from build123d import *

# Parameters (mm, degrees)
F2_R = 5
F4_D = 11


with BuildPart() as f1:
    # F0 (on Front) → F1 (revolve)
    with BuildSketch(Plane.XZ):
        Polygon((0, 101), (0, 32), (10, 32), (10, 55), (32, 55), (32, 70), (20, 70), (20, 101), align=None)
    revolve(axis=Axis((86.927190423, 0, 0), (1, 0, 0)))

    # F2
    f2_edges = [f1.edges().sort_by_distance(p)[0] for p in [
        (20, 0, -70),
    ]]
    fillet(f2_edges, radius=F2_R)

    # F4 (through all)
    with Locations(Plane.YZ.offset(20)):
        with Locations((46.25, 80.1073498501), (-92.5, 0), (46.25, -80.1073498501)):
            Hole(F4_D / 2)


solid = f1.part
Source: CAD feature listing. Evaluate the final solid. Frame: model axes, mm. A direction names the side the tool comes from. Coordinates: 2 decimals unless noted, no trailing zeros. Loops run counter-clockwise (first coordinate to the right, second up) from the corner with the lowest first, then second, coordinate; pieces in that order, holes last. Notation, with made-up numbers: (-38.5, 52) - (-28.5, 52) arc R18 cw to (-28.5, 84) - close; hole circle Ø1 at (76, 35.25). An arc over 180 degrees is marked (long way). Return JSON: item names as keys, results as strings.
Q1. Section D-D, the plane x = 29.5. Return loops of the section in (y, z).
Results:
{"outline": "circle Ø140 at (0, 0); hole circle Ø110 at (0, 0)"}
Q2. Section C-C, the plane z = -83. Return loops of the section in (x, y), plus the area to 3 significant figures.
Results:
{"outline": "(0, -57.55) - (20, -57.55) - (20, 41.57) - (0, 41.57) - close; (0, 50.93) - (20, 50.93) - (20, 57.55) - (0, 57.55) - close", "area": "2,110 mm2"}
Q3. Material intervals for line 1 along Y through (x, z) = (30, 0.5); line 2 along Z through (x, y) = (5, 0); line 3 along X through (y, z) = (7, 38.5), sorted ascending.
Results:
{"line 1": "-70 to -55, 55 to 70", "line 2": "-101 to -32, 32 to 101", "line 3": "0 to 10"}
Q4. Access query for faces 4 (the flat face through (20, 67, 38)), 5 (the flat face through (32, 36, 42)). Directions: +Z, -Z, +X, -X, +Y, -Y. A direction counts if a zero-diameter tool reaches every point of the face in a straight line with its end or side. Return the directions, or none.
Results:
{"face 4": "+X", "face 5": "+Z, -Z, +X, +Y, -Y"}
Q5. Section A-A, the plane y = 0. Return loops of the section in (x, z).
Results:
{"outline": "(0, -101) - (20, -101) - (20, -75) arc R5 cw to (25, -70) - (32, -70) - (32, -55) - (10, -55) - (10, -32) - (0, -32) - close; (0, 32) - (10, 32) - (10, 55) - (32, 55) - (32, 70) - (25, 70) arc R5 cw to (20, 75) - (20, 101) - (0, 101) - close"}
Q6. Contact query for flat-ended pins moving along their axis: P1, Ø3, axis at x = 20, z = -3, coming from the -Y side; P2, Ø6, axis at x = 17, y = 12, coming from the -Z side; P3, Ø10, axis at x = 7.5, y = 71, coming from the -Z side; P4, Ø12, axis at y = -31.5, z = -43, coming from the +X side. Output: stop coordinate, or through.
Results:
{"P1": "y = -100.99", "P2": "z = -100.6", "P3": "z = -76.45", "P4": "x = 32"}
Q7. Mould query, pull axis Z, two halves, no side actions, for faces 1 (the cylindrical face through (21.154, 53.692, -11.923)), 2 (the cylindrical face through (9.86, 98.6, -21.89)), 3 (the flat face through (0, -24, -24)). Classes: released by +Z, released by -Z, zero draft, split by the parting line, or undercut.
Results:
{"face 1": "undercut", "face 2": "split by the parting line", "face 3": "zero draft"}
Q8. Section B-B, the plane z = 0. Return loops of the section in (x, y).
Results:
{"outline": "(0, -101) - (20, -101) - (20, -98) - (0, -98) - close; (0, -87) - (20, -87) - (20, -75) arc R5 cw to (25, -70) - (32, -70) - (32, -55) - (10, -55) - (10, -32) - (0, -32) - close; (0, 32) - (10, 32) - (10, 55) - (32, 55) - (32, 70) - (25, 70) arc R5 cw to (20, 75) - (20, 101) - (0, 101) - close"}
